Source: CAD feature listing. Evaluate the final solid. Frame: model axes, mm. Give positions to 0.01 mm unless a question says otherwise; leave off trailing zeros. Order: outer loops, then holes, each group sorted by start corner. A loop starts at its lowest first (then second) coordinate and runs counter-clockwise, first axis right, second up. Notation, with made-up numbers: M 3.25,-23 L 37.25,-23 A19 ccw 37.25,-2 Z; hole C 83.5,-4.75 d3. An arc over 180 degrees is marked long. Answer in a Markdown table with one row per item. Add a question column.
(1) Section query A-A, the plane z = 42.65. Return loops of the section in (x, y), plus the area to 3 significant figures.
(2) Section query D-D, the plane x = 22.5. Return loops of the section in (y, z).
(3) Pin query (flat end, axial travel): P1, Ø2.5, axis at x = 9.15, z = 42.65, coming from the -Y side. Return the tip coordinate at first contact, or that it passes through.
(4) Section query C-C, the plane z = 18. Return loops of the section in (x, y).
(5) Section query B-B, the plane x = 9.15. Return loops of the section in (y, z), plus the area to 3 significant figures.
(6) Material intervals for line 1 along Z through (x, y) = (8, 1.25); line 2 along Z through (x, y) = (8.5, 1.9); line 3 along Z through (x, y) = (9.5, 0.35), sorted ascending.
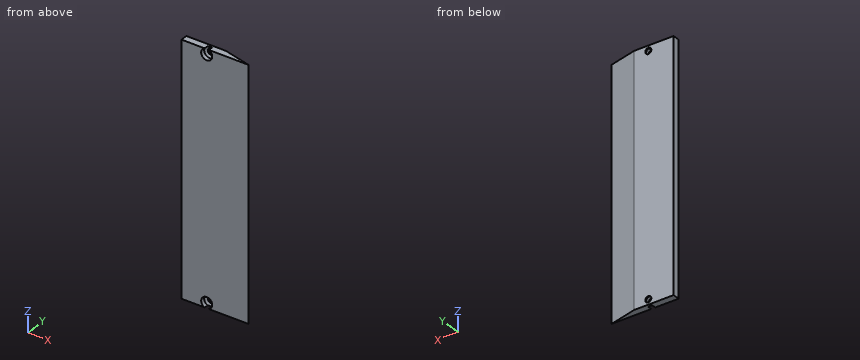
from build123d import *

# Parameters (mm, degrees)
BOSS_EXTRUDE1_DEPTH = 44.5
HOLEWZD2_AT_2_COUNT = 2
HOLEWZD2_AT_2_PITCH = 85.3


with BuildPart() as part:
    # Sketch1 → Boss-Extrude1 (new, symmetric)
    with BuildSketch(Plane.XY):
        Polygon((0, 0), (0, 2.5), (14.273047666, 2.5), (24.3, 0), align=None)
    extrude(amount=BOSS_EXTRUDE1_DEPTH, both=True)

    # Sketch6 → HoleWzd2 (revolve, cut)
    with BuildSketch(Plane(origin=(9.15, 0, 42.65), x_dir=(0, 0, -1), z_dir=(1, 0, 0))):
        Polygon((0, 0), (0, 2.5), (1.1, 2.5), (1.1, 2.040774557), (2, 1.5), (2, 0), align=None)
    holewzd2 = revolve(axis=Axis((9.15, -6.130023899, 42.65), (0, 1, 0)), mode=Mode.SUBTRACT)

    # HoleWzd2 at 2: HoleWzd2 ×2
    with Locations(*[(0, 0, -i * HOLEWZD2_AT_2_PITCH) for i in range(1, HOLEWZD2_AT_2_COUNT)]):
        add(holewzd2, mode=Mode.SUBTRACT)


solid = part.part
Values follow:
| question | item | result |
|---|---|---|
| 1 | outline | M 0,0 L 7.15,0 L 7.15,1.5 L 8.05,2.04 L 8.05,2.5 L 0,2.5 Z; M 10.25,2.04 L 11.15,1.5 L 11.15,0 L 24.3,0 L 14.27,2.5 L 10.25,2.5 Z |
| 1 | area | 39.5 mm² |
| 2 | outline | M 0,-44.5 L 0.45,-44.5 L 0.45,44.5 L 0,44.5 Z |
| 3 | P1 | stops at y = 1.95 |
| 4 | outline | M 0,0 L 24.3,0 L 14.27,2.5 L 0,2.5 Z |
| 5 | outline | M 0,-40.65 L 1.5,-40.65 L 2.04,-41.55 L 2.5,-41.55 L 2.5,41.55 L 2.04,41.55 L 1.5,40.65 L 0,40.65 Z; M 1.59,-44.5 L 2.5,-44.5 L 2.5,-43.75 L 2.04,-43.75 Z; M 1.59,44.5 L 2.04,43.75 L 2.5,43.75 L 2.5,44.5 Z |
| 5 | area | 206 mm² |
| 6 | line 1 | z = -44.5 to -44.29, -41.01 to 41.01, 44.29 to 44.5 |
| 6 | line 2 | z = -44.5 to -43.82, -41.48 to 41.48, 43.82 to 44.5 |
| 6 | line 3 | z = -40.68 to 40.68 |
